from build123d import *

# Parameters (mm, degrees)
SKETCH_1_R      = 0.75
EXTRUDE_1_DEPTH = 2.9


with BuildPart() as part:
    # 草图1 → 凸台-拉伸1 (new body)
    with BuildSketch(Plane.XY):
        with BuildLine():
            Line((-10.5, 22.5), (-10.5, 13.638181697))
            ThreePointArc((-10.5, 13.638181697), (-7.5, 0), (-10.5, -13.638181697))
            Line((-10.5, -13.638181697), (-10.5, -22.5))
            ThreePointArc((-10.5, -22.5), (0, -33), (10.5, -22.5))
            Line((10.5, -22.5), (10.5, -13.638181697))
            ThreePointArc((10.5, -13.638181697), (7.5, 0), (10.5, 13.638181697))
            Line((10.5, 13.638181697), (10.5, 22.5))
            ThreePointArc((10.5, 22.5), (0, 33), (-10.5, 22.5))
        make_face()
        with Locations((6, 28.25)):
            Circle(SKETCH_1_R, mode=Mode.SUBTRACT)
        with Locations((-6, 28.25)):
            Circle(SKETCH_1_R, mode=Mode.SUBTRACT)
        with Locations((6, -28.25)):
            Circle(SKETCH_1_R, mode=Mode.SUBTRACT)
        with Locations((-6, -28.25)):
            Circle(SKETCH_1_R, mode=Mode.SUBTRACT)
        with BuildLine():
            ThreePointArc((4, 22.500000371), (-3.71e-07, 26.5), (-4, 22.499999629))
            Line((-4, 22.499999629), (-4, 8.5))
            Line((-4, 8.5), (4, 8.5))
            Line((4, 8.5), (4, 22.500000371))
        make_face(mode=Mode.SUBTRACT)
        with BuildLine():
            Line((4, -22.500000371), (4, -8.5))
            Line((4, -8.5), (-4, -8.5))
            Line((-4, -8.5), (-4, -22.499999629))
            ThreePointArc((-4, -22.499999629), (-3.71e-07, -26.5), (4, -22.500000371))
        make_face(mode=Mode.SUBTRACT)
    extrude(amount=EXTRUDE_1_DEPTH)


solid = part.part
Build history of the part. All positions in model axes, mm. A direction names the side the tool comes from. Round coordinates to 2 decimals unless told otherwise and drop trailing zeros. Write each loop counter-clockwise with the first axis right and the second up, starting at its lowest first coordinate (ties: lowest second). Pieces come first, ordered by that corner, then holes. Notation, with made-up numbers: (-10, -14) -> (31, -14) arc R13 ccw to (31, 9) -> close; hole circle Ø1 at (63, 20.25). An arc over 180 degrees is marked (long way). Use one line per item in the form item = value.
Q1. Drop flat-ended pins along their axis: P1, Ø0.9, axis at y = 13, z = 1.5, coming from the -X side; P2, Ø1.2, axis at x = -6, y = -28.25, coming from the -Z side; P3, Ø1.5, axis at y = -3.5, z = 0.5, coming from the -X side. Give the stop position or say it passes through.
Conclusion:
P1 = -10.41
P2 = through
P3 = -7.78
Q2. Band-saw the part on D-D, the plane y = -28.25. Write the cut outline in (x, z), then the cut area to 3 significant figures.
Conclusion:
outline = (-8.79, 0) -> (-6.75, 0) -> (-6.75, 2.9) -> (-8.79, 2.9) -> close; (-5.25, 0) -> (5.25, 0) -> (5.25, 2.9) -> (-5.25, 2.9) -> close; (6.75, 0) -> (8.79, 0) -> (8.79, 2.9) -> (6.75, 2.9) -> close
area = 42.3 mm²
Q3. Drill centre lines: L1, parallel to Y at x = -0.25, z = 2.4; L2, parallel to Y at x = -2, z = 1.2; L3, parallel to X at y = -16.5, z = 2.75. Where is each one in solid material? Low to high.
Conclusion:
L1 = -33 to -26.49, -8.5 to 8.5, 26.49 to 33
L2 = -32.81 to -25.96, -8.5 to 8.5, 25.96 to 32.81
L3 = -10.5 to -4, 4 to 10.5
Q4. Tool access for faces 4 (the flat face through (4, -16, 1)), 5 (the cylindrical face through (-7.5, 0.2, 1.4)): list every direction of +Z, -Z, +X, -X, +Y, -Y with a clear straight run to the whole face (end or side of a thin tool).
Conclusion:
face_4 = +Z, -Z
face_5 = +Z, -Z, -X
Q5. Two-plate mould, pull along X, no slides. Class faces 1 (the flat face through (0, 0, 2.9)), 2 (the flat face through (0, 8.5, 1)), 3 (the flat face through (10.5, -18, 1)): released by +X, released by -X, zero draft, split by the parting line, or undercut.
Conclusion:
face_1 = zero draft
face_2 = undercut
face_3 = released by +X
Q6. Band-saw the part on B-B, the plane z = 2. Write the cut outline in (x, y), then the cut area to 3 significant figures.
Conclusion:
outline = (-10.5, -22.5) arc R10.5 ccw to (10.5, -22.5) -> (10.5, -13.64) arc R32.5 cw to (10.5, 13.64) -> (10.5, 22.5) arc R10.5 ccw to (-10.5, 22.5) -> (-10.5, 13.64) arc R32.5 cw to (-10.5, -13.64) -> close; hole circle Ø1.5 at (-6, -28.25); hole circle Ø1.5 at (-6, 28.25); hole (-4, -22.5) arc R4 ccw to (4, -22.5) -> (4, -8.5) -> (-4, -8.5) -> close; hole (-4, 8.5) -> (4, 8.5) -> (4, 22.5) arc R4 ccw to (-4, 22.5) -> close; hole circle Ø1.5 at (6, -28.25); hole circle Ø1.5 at (6, 28.25)
area = 900 mm²
Q7. Band-saw the part on A-A, the plane y = -21.5. Write the cut outline in (x, z).
Conclusion:
outline = (-10.5, 0) -> (-4, 0) -> (-4, 2.9) -> (-10.5, 2.9) -> close; (4, 0) -> (10.5, 0) -> (10.5, 2.9) -> (4, 2.9) -> close
Q8. Band-saw the part on C-C, the plane x = 2.5. Write the cut outline in (y, z), then the cut area to 3 significant figures.
Conclusion:
outline = (-32.7, 0) -> (-25.62, 0) -> (-25.62, 2.9) -> (-32.7, 2.9) -> close; (-8.5, 0) -> (8.5, 0) -> (8.5, 2.9) -> (-8.5, 2.9) -> close; (25.62, 0) -> (32.7, 0) -> (32.7, 2.9) -> (25.62, 2.9) -> close
area = 90.3 mm²
